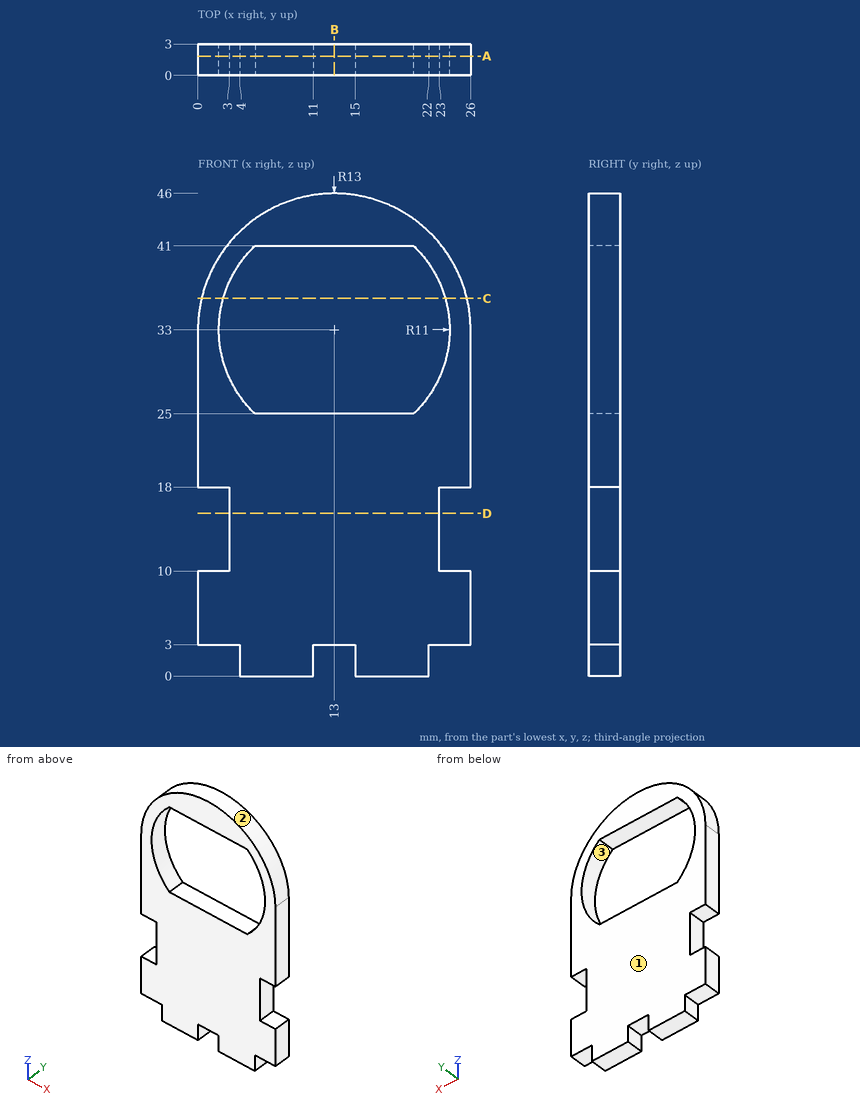
Input: dimensioned drawing with shaded views. Units: mm. Origin: part minimum x, y, z. Give positions to 0.01 mm unless a question says otherwise; leave off trailing zeros. Write each loop counter-clockwise with the first axis right and the second up, starting at its lowest first coordinate (ties: lowest second). Pieces come first, ordered by that corner, then holes.
1. Section query C-C (z = 36). Return the cut outline in (x, y).
2. Pull-direction query (Z, two-part tool) for the marked faces 1, 2 and 3; classes: +Z half, -Z half, draft (parallel to the pull), parting line (faces both ways), or undercut.
3. First-contact query: pin 1 (0.9 mm diameter, centred on x = 11, y = 1.5, fed in from +Z); pin 2 (1.5 mm diameter, centred on y = 1, z = 1, fed in from -X); pin 3 (1.5 mm diameter, centred on y = 1.5, z = 15.5, fed in from +X); pin 4 (1 mm diameter, centred on y = 2, z = 8, fed in from -X). Flat tips, straight axial feed; report the tip coordinate or a pass-through.
4. Section query A-A (y = 1.85). Return the cut outline in (x, z).
5. Material intervals for line 1 along Z through (x, y) = (12.75, 1.95); line 2 along Z through (x, y) = (20.25, 0.55); line 3 along X through (y, z) = (0.65, 40.5), sorted ascending.
6. Section query D-D (z = 15.5). Return the cut outline in (x, y).
7. Section query B-B (x = 13). Return the cut outline in (y, z), then the cut area to 3 significant figures.
Output values:
1. outline: (0.35, 0) - (2.42, 0) - (2.42, 3) - (0.35, 3) - close; (23.58, 0) - (25.65, 0) - (25.65, 3) - (23.58, 3) - close
2. face 1: draft
2. face 2: +Z half
2. face 3: undercut
3. pin 1: stops at z = 45.91
3. pin 2: stops at x = 4
3. pin 3: stops at x = 23
3. pin 4: stops at x = 0
4. outline: (0, 3) - (4, 3) - (4, 0) - (11, 0) - (11, 3) - (15, 3) - (15, 0) - (22, 0) - (22, 3) - (26, 3) - (26, 10) - (23, 10) - (23, 18) - (26, 18) - (26, 33) arc R13 ccw to (0, 33) - (0, 18) - (3, 18) - (3, 10) - (0, 10) - close; hole (5.45, 25) - (20.55, 25) arc R11 ccw to (20.55, 41) - (5.45, 41) arc R11 ccw to start
5. line 1: z = 3 to 25, 41 to 46
5. line 2: z = 0 to 25, 41 to 43.79
5. line 3: x = 2.38 to 4.95, 21.05 to 23.62
6. outline: (3, 0) - (23, 0) - (23, 3) - (3, 3) - close
7. outline: (0, 3) - (3, 3) - (3, 25) - (0, 25) - close; (0, 41) - (3, 41) - (3, 46) - (0, 46) - close
7. area: 81.0 mm2
